Autodesk Inventor part; units mm, degrees
ref_plane "bolt_XY" through (20, 0, 0) normal (1, 0, 0) x (0, 0, -1)
ref_plane "bolt_YZ" through (20, 0, 0) normal (0, 0, -1) x (0, 1, 0)
ref_plane "bolt_ZX" through (20, 0, 0) normal (0, 1, 0) x (1, 0, 0)
sketch "Sketch_1" plane through (0, 0, 0) normal (0, 0, 1) x (1, 0, 0)
  line L0 (20, 0) -> (-5, 0)
  line L1 (-5, 0) -> (-5, 3.75)
  line L2 (-5, 3.75) -> (-4.5, 4.25)
  line L3 (-4.5, 4.25) -> (0, 4.25)
  line L4 (0, 4.25) -> (0, 2.5)
  line L5 (0, 2.5) -> (19.5095, 2.5)
  line L6 (19.5095, 2.5) -> (20, 2.0095)
  line L7 (20, 2.0095) -> (20, 0)
  line L8 (20, 0) -> (-5, 0)
revolve "Revolution1" add sketch "Sketch_1" angle 360 about axis through (20, 0, 0) along (1, 0, 0)
thread "Thread1"
sketch "Sketch2" plane through (-5, 0, 0) normal (-1, 0, 0) x (0, 0, 1)
  point P0 (0, 0)
hole "Hole1" at (-5, 0, 0) direction (1, 0, 0) diameter 4 depth 2.5 tip angle 120
sketch "Sketch_3" plane through (-5, 0, 0) normal (1, 0, 0) x (0, 0, -1)
  line L0 (-2, -1.1547) -> (0, -2.3094)
  line L1 (0, -2.3094) -> (2, -1.1547)
  line L2 (2, -1.1547) -> (2, 1.1547)
  line L3 (2, 1.1547) -> (0, 2.3094)
  line L4 (0, 2.3094) -> (-2, 1.1547)
  line L5 (-2, 1.1547) -> (-2, -1.1547)
extrude "Extrusion1" cut sketch "Sketch_3" along normal blind 2.5
ref_plane "bolt_XY" through (20, 0, 0) normal (1, 0, 0) x (0, 0, -1)
ref_plane "bolt_YZ" through (20, 0, 0) normal (0, 0, -1) x (0, 1, 0)
ref_plane "bolt_ZX" through (20, 0, 0) normal (0, 1, 0) x (1, 0, 0)
ref_plane "nut_XY" through (0, 0, 0) normal (1, 0, 0) x (0, 0, -1)
ref_plane "nut_YZ" through (0, 0, 0) normal (0, 0, -1) x (0, 1, 0)
ref_plane "nut_ZX" through (0, 0, 0) normal (0, 1, 0) x (1, 0, 0)
properties part number "CBE5-20"
Read the model definition and answer for the solid it produces. Units are mm, in the model's axes. A direction names the side the tool comes from. Coordinates: 2 decimals unless noted, no trailing zeros. Write each loop counter-clockwise with the first axis right and the second up, starting at its lowest first coordinate (ties: lowest second). Pieces come first, ordered by that corner, then holes. Notation, with made-up numbers: (69.5, 67.25) -> (92.5, 67.25) arc R19 ccw to (92.5, 83.25) -> close; hole circle Ø6 at (38.25, 2). An arc over 180 degrees is marked (long way). Return JSON: item names as keys, results as strings.
(1) The part is cut by section A-A on x = 14.75. Give the vertices of the cut face in (y, z), then the cut area to 3 significant figures.
Answers below:
{"outline": "circle Ø5 at (0, 0)", "area": "19.6 mm^2"}
(2) Which of the six approach directions +Z, -Z, +X, -X, +Y, -Y give full straight-line access (tool end or side, diameter ignored) to faces 1 (the flat face through (-3.77, 1.74, 0.99)), 2 (the flat face through (20, 0, 0)), 3 (the cylindrical face through (9.89, -0.54, -2.44))?
Answers below:
{"face 1": "-X", "face 2": "+Z, -Z, +X, +Y, -Y", "face 3": "+X"}
(3) Consider line 1 along X through (y, z) = (-1.75, -2); line 2 along Z through (x, y) = (14, 0); line 3 along X through (y, z) = (-0.5, -1.25). Determine where each line is inside the solid, lowest interval first. Write a range as from..to.
Answers below:
{"line 1": "-5..0", "line 2": "-2.5..2.5", "line 3": "-2.12..20"}
(4) Each of these flat-tipped pins is pushed along its axis until it touches: P1, Ø1.5, axis at x = 6.5, y = -1, coming from the -Z side; P2, Ø0.5, axis at y = 1, z = 1.5, coming from the -X side; P3, Ø1.5, axis at x = 6, z = -1.5, coming from the +Y side; P4, Ø3, axis at y = -3, z = 2.5, coming from the -X side. Where does it stop, or does it pass through?
Answers below:
{"P1": "z = -2.49", "P2": "x = -2.5", "P3": "y = 2.38", "P4": "x = -5"}
